```python
from build123d import *

# Parameters (mm, degrees)
F1_DEPTH = 2000


with BuildPart() as f1:
    # F0 (on Front) → F1 (new body)
    with BuildSketch(Plane.XZ):
        with BuildLine():
            Line((-25.322348, 0), (0, 0))
            Line((0, 0), (25.322348, 0))
            ThreePointArc((25.322348, 0), (28.919047, 1.526708), (30.319303, 5.174497))
            Line((30.319303, 5.174497), (28.371131, 60.96284))
            Line((28.371131, 60.96284), (27.385817, 60.524813))
            Line((27.385817, 60.524813), (29.319912, 5.139598))
            ThreePointArc((29.319912, 5.139598), (28.199708, 2.221367), (25.322348, 1))
            Line((25.322348, 1), (0, 1))
            Line((0, 1), (-25.322348, 1))
            ThreePointArc((-25.322348, 1), (-28.199708, 2.221367), (-29.319912, 5.139598))
            Line((-29.319912, 5.139598), (-27.385817, 60.524813))
            Line((-27.385817, 60.524813), (-28.371131, 60.96284))
            Line((-28.371131, 60.96284), (-30.319303, 5.174497))
            ThreePointArc((-30.319303, 5.174497), (-28.919047, 1.526708), (-25.322348, 0))
        make_face()
    extrude(amount=-F1_DEPTH)


solid = f1.part
```
Model file for the job. Use its own axes, mm. Give positions to 0.01 mm unless a question says otherwise; leave off trailing zeros. Order: outer loops, then holes, each group sorted by start corner. A loop starts at its lowest first (then second) coordinate and runs counter-clockwise, first axis right, second up.
1) Saw through at B-B, the plane y = 267. Write the cut outline in (x, z).
2) Pin check, flat tips, straight feed: pin 1 (8 mm diameter, centred on y = 1315, z = 33.5, fed in from -X); pin 2 (4 mm diameter, centred on x = -15.5, y = 449, fed in from +Z); pin 3 (12 mm diameter, centred on y = 1477, z = 20.5, fed in from +X). Stop position of each tip, or through.
3) Mould opens along X. For faces 1 (the flat face through (0, 986, 1)), 2 (the flat face through (-29, 0, 19)) say: +X half, -X half, draft (parallel to the pull), parting line (faces both ways), or undercut.
4) Wall check: probe 1 along X at (y, z) = (484, 54.5); probe 2 along X at (y, z) = (714, 50); probe 3 along Z at (x, y) = (-15.5, 870). Give the ranges that are in metal, low to high.
5) Saw through at A-A, the plane z = 49. Write the cut outline in (x, y), then the cut area to 3 significant figures.
6) Saw through at C-C, the plane x = -14.5. Write the cut outline in (y, z).
Computed:
1. outline: (-30.32, 5.17) arc R5 ccw to (-25.32, 0) - (25.32, 0) arc R5 ccw to (30.32, 5.17) - (28.37, 60.96) - (27.39, 60.52) - (29.32, 5.14) arc R4 cw to (25.32, 1) - (-25.32, 1) arc R4 cw to (-29.32, 5.14) - (-27.39, 60.52) - (-28.37, 60.96) - close
2. pin 1: stops at x = -29.47
2. pin 2: stops at z = 1
2. pin 3: stops at x = 29.99
3. face 1: undercut
3. face 2: draft
4. probe 1: x = -28.6 to -27.6, 27.6 to 28.6
4. probe 2: x = -28.75 to -27.75, 27.75 to 28.75
4. probe 3: z = 0 to 1
5. outline: (-28.79, 0) - (-27.79, 0) - (-27.79, 2000) - (-28.79, 2000) - close; (27.79, 0) - (28.79, 0) - (28.79, 2000) - (27.79, 2000) - close
5. area: 4,000 mm2
6. outline: (0, 0) - (2000, 0) - (2000, 1) - (0, 1) - close
